```python
from build123d import *

# Parameters (mm, degrees)
SKETCH1_W               = 72
SKETCH1_H               = 23.7
BOSS_EXTRUDE1_DEPTH     = 12
SKETCH3_W               = 23.7
SKETCH3_H               = 7.8
BOSS_EXTRUDE2_DEPTH     = 8.1
SKETCH2_R               = 2.45
CUT_EXTRUDE1_DEPTH      = 60
CUT_EXTRUDE2_DEPTH      = 43.871931377
CUT_EXTRUDE2_DEPTH_BACK = 43.871931377
SKETCH4_R               = 2.5


with BuildPart() as part:
    # Sketch1 → Boss-Extrude1 (new, symmetric)
    with BuildSketch(Plane.XY):
        Rectangle(SKETCH1_W, SKETCH1_H)
    extrude(amount=BOSS_EXTRUDE1_DEPTH, both=True)

    # Sketch3 → Boss-Extrude2 (add)
    with BuildSketch(Plane(origin=(0, 11.85, 0), x_dir=(1, 0, 0), z_dir=(0, 1, 0))):
        with Locations((16.15, -8.1)):
            Rectangle(SKETCH3_W, SKETCH3_H)
        with Locations((16.15, 8.1)):
            Rectangle(SKETCH3_W, SKETCH3_H)
    extrude(amount=BOSS_EXTRUDE2_DEPTH)

    # Sketch2 → Cut-Extrude1 (cut)
    with BuildSketch(Plane(origin=(36, 0, 0), x_dir=(0, 0, -1), z_dir=(1, 0, 0))):
        with Locations((0, -0.3)):
            Circle(SKETCH2_R)
    extrude(amount=-CUT_EXTRUDE1_DEPTH, mode=Mode.SUBTRACT)

    # Sketch4 → Cut-Extrude2 (cut, two sides: drawn at the far end of the back side and taken through both)
    with BuildSketch(Plane.XY.offset(-CUT_EXTRUDE2_DEPTH_BACK)):
        with Locations((8.3, 16.05)):
            Circle(SKETCH4_R)
        with Locations((23.9, 16.05)):
            Circle(SKETCH4_R)
    extrude(amount=CUT_EXTRUDE2_DEPTH + CUT_EXTRUDE2_DEPTH_BACK, mode=Mode.SUBTRACT)


solid = part.part
```
Verification items for the finished model (mm, model axes). A direction names the side the tool comes from. Round coordinates to 2 decimals unless told otherwise and drop trailing zeros. Order: outer loops, then holes, each group sorted by start corner. A loop starts at its lowest first (then second) coordinate and runs counter-clockwise, first axis right, second up.
1) Material ranges on line 1 (X direction, y = 16.05, z = -6.5); line 2 (Y direction, x = 23.5, z = 0.25); line 3 (Y direction, x = 23.9, z = -8.75), recorded low to high.
Geometry says:
line 1: x = 4.3 to 5.8, 10.8 to 21.4, 26.4 to 28
line 2: y = -11.85 to -2.74, 2.14 to 11.85
line 3: y = -11.85 to 13.55, 18.55 to 19.95
2) Cross-section at B-B, the plane y = 16.05. Record the cut outline in (x, z).
Geometry says:
outline: (4.3, -12) - (5.8, -12) - (5.8, -4.2) - (4.3, -4.2) - close; (4.3, 4.2) - (5.8, 4.2) - (5.8, 12) - (4.3, 12) - close; (10.8, -12) - (21.4, -12) - (21.4, -4.2) - (10.8, -4.2) - close; (10.8, 4.2) - (21.4, 4.2) - (21.4, 12) - (10.8, 12) - close; (26.4, -12) - (28, -12) - (28, -4.2) - (26.4, -4.2) - close; (26.4, 4.2) - (28, 4.2) - (28, 12) - (26.4, 12) - close
3) Cross-section at A-A, the plane x = 8.3. Record the cut outline in (y, z), plus the area to 3 significant figures.
Geometry says:
outline: (-11.85, -12) - (13.55, -12) - (13.55, -4.2) - (11.85, -4.2) - (11.85, 4.2) - (13.55, 4.2) - (13.55, 12) - (-11.85, 12) - close; (18.55, -12) - (19.95, -12) - (19.95, -4.2) - (18.55, -4.2) - close; (18.55, 4.2) - (19.95, 4.2) - (19.95, 12) - (18.55, 12) - close; hole circle Ø4.9 at (-0.3, 0)
area: 598 mm2
4) Depth check by flat-ended pin: pin 1 (6 mm diameter, centred on y = 15.5, z = 8.5, fed in from +X); pin 2 (2.5 mm diameter, centred on y = 17.5, z = -6, fed in from -X); pin 3 (2.5 mm diameter, centred on y = 0, z = -0.5, fed in from +X). Enter the tip coordinate at first touch or a pass-through.
Geometry says:
pin 1: stops at x = 28
pin 2: stops at x = 4.3
pin 3: stops at x = -24
5) Cross-section at D-D, the plane x = -1. Record the cut outline in (y, z).
Geometry says:
outline: (-11.85, -12) - (11.85, -12) - (11.85, 12) - (-11.85, 12) - close; hole circle Ø4.9 at (-0.3, 0)
6) Tool access check on faces 5 (the flat face through (4.3, 16, -8)), 6 (the flat face through (28, 16, 8)), 7 (the flat face through (16, 16, -4.2)). Record the directions out of +Z, -Z, +X, -X, +Y, -Y that give a thin tool (end or side, any length) a straight path to the whole face; none if there is none.
Geometry says:
face 5: +Z, -Z, -X, +Y
face 6: +Z, -Z, +X, +Y
face 7: +X, -X, +Y
7) Draft check along X on faces 1 (the flat face through (28, 16, -8)), 2 (the cylindrical face through (26.21, 15.09, 8.05)), 3 (the cylindrical face through (9.45, 13.83, -8.15)), 4 (the cylindrical face through (6.4, -2.7, 0.5)). Enter one of: +X half, -X half, draft (parallel to the pull), parting line (faces both ways), or undercut.
Geometry says:
face 1: +X half
face 2: undercut
face 3: undercut
face 4: draft
8) Cross-section at C-C, the plane z = 0. Record the cut outline in (x, y), plus the area to 3 significant figures.
Geometry says:
outline: (-36, -11.85) - (36, -11.85) - (36, -2.75) - (-24, -2.75) - (-24, 2.15) - (36, 2.15) - (36, 11.85) - (-36, 11.85) - close
area: 1,410 mm2
